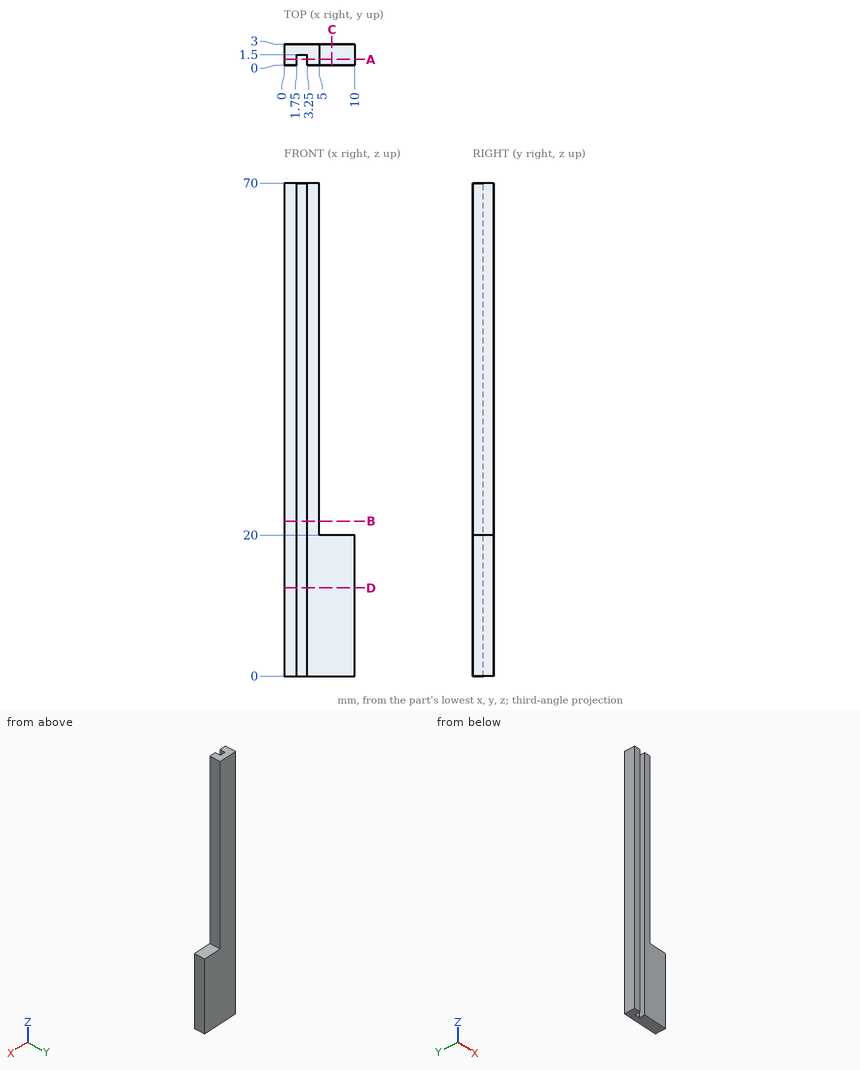
Can you work these out from the drawing? Everything is in mm from the part's minimum corner. Give positions to 0.01 mm unless a question says otherwise; leave off trailing zeros. Order: outer loops, then holes, each group sorted by start corner. A loop starts at its lowest first (then second) coordinate and runs counter-clockwise, first axis right, second up. Notation, with made-up numbers: M -27,-18 L 32,-18 A25 ccw 32,1 Z; hole C 27,-35.75 d5. An arc over 180 degrees is marked long. Write item = value, one per line. Start each with the question number.
Q1. Suppose I cut it at D-D (z = 12.5). Write out the boundary of the cut face in (x, y).
Q2. Suppose I cut it at C-C (x = 6.75). Write out the boundary of the cut face in (y, z), plus the area to 3 significant figures.
Q3. Suppose I cut it at B-B (z = 22). Write out the boundary of the cut face in (x, y).
Q4. I need wall thicknesses on probe 1 along X at (y, z) = (0.3, 52.5); probe 2 along X at (y, z) = (1.15, 11.5); probe 3 along X at (y, z) = (2.2, 67). Which ranges of each line are inside material? Lowest first, please. Write a range as [from, to].
Q5. Will this pin go through, and if not, where does the flat tip stop? pin 1 Ø1.5 at (y, z) = (1.5, 61.5) entering from +X.
Q6. Suppose I cut it at A-A (y = 0.8). Write out the boundary of the cut face in (x, z), plus the area to 3 significant figures.
Check result:
q1.outline = M 0,0 L 1.75,0 L 1.75,1.5 L 3.25,1.5 L 3.25,0 L 10,0 L 10,3 L 0,3 Z
q2.outline = M 0,0 L 3,0 L 3,20 L 0,20 Z
q2.area = 60.0 mm2
q3.outline = M 0,0 L 1.75,0 L 1.75,1.5 L 3.25,1.5 L 3.25,0 L 5,0 L 5,3 L 0,3 Z
q4.probe_1 = [0, 1.75], [3.25, 5]
q4.probe_2 = [0, 1.75], [3.25, 10]
q4.probe_3 = [0, 5]
q5.pin_1 = 5
q6.outline = M 0,0 L 1.75,0 L 1.75,70 L 0,70 Z; M 3.25,0 L 10,0 L 10,20 L 5,20 L 5,70 L 3.25,70 Z
q6.area = 345 mm2
